The drawing under review shows one solid part. Ordinate dimensions are in mm from its lowest x, y, z. A direction names the side the tool comes from. Coordinates: 2 decimals unless noted, no trailing zeros. Write each loop counter-clockwise with the first axis right and the second up, starting at its lowest first coordinate (ties: lowest second). Pieces come first, ordered by that corner, then holes. Notation, with made-up numbers: M -38.5,-6 L -2.5,-6 A17 ccw -2.5,1 Z; hole C 62.25,52 d3. An arc over 180 degrees is marked long. Write item = value, one per line.
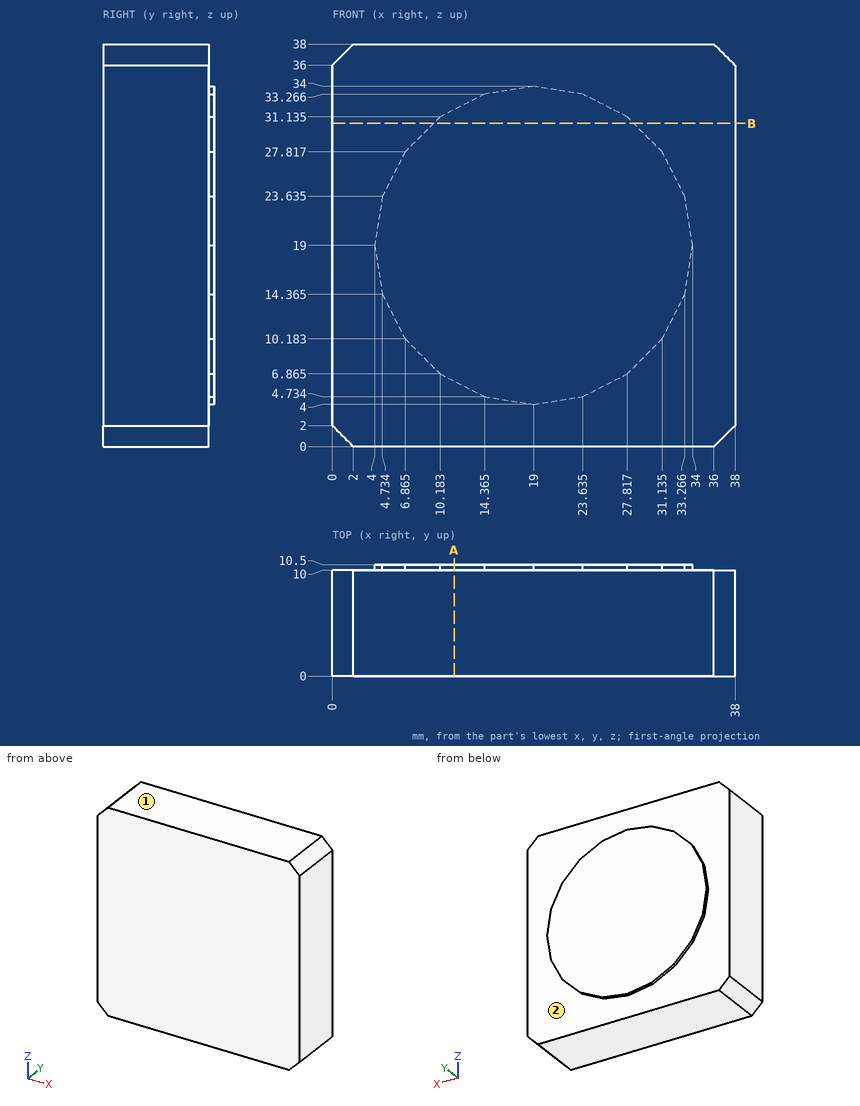
Q1. Machinability: for the marked faces 1 and 2, which of the approach directions +Z, -Z, +X, -X, +Y, -Y give a long, thin tool a straight path to every point of the face, cutting with its end or side? Answer none if there is none.
Check result:
face_1 = +Z, +X, -X, +Y, -Y
face_2 = +Y
Q2. Wall thickness on line 1 (Y direction, x = 36.5, z = 12.5): over which ranges is the line inside the solid? List them lowest first.
Check result:
line_1 = 0 to 10
Q3. Consider section A-A, the plane x = 11.5. State the section outline as (y, z) points, and give its area (3 significant figures).
Check result:
outline = M 0,0 L 10,0 L 10,6.19 L 10.5,6.19 L 10.5,31.81 L 10,31.81 L 10,38 L 0,38 Z
area = 393 mm²
Q4. Consider section B-B, the plane z = 30.5. State the section outline as (x, y) points.
Check result:
outline = M 0,0 L 38,0 L 38,10 L 28.45,10 L 28.45,10.5 L 9.55,10.5 L 9.55,10 L 0,10 Z
